from build123d import *

# Parameters (mm, degrees)
F0_R     = 45
F0_R_2   = 30.25
F1_DEPTH = 50
F2_R     = 80
F2_R_2   = 5
F3_DEPTH = 20
F4_R     = 26
F4_R_2   = 21
F5_DEPTH = 30
F6_SIZE2 = 40
F6_SIZE  = 10
F7_R     = 2
F8_DEPTH = 85
F9_R     = 3


with BuildPart() as f1:
    # F0 (on Top) → F1 (new body)
    with BuildSketch(Plane.XY):
        Circle(F0_R)
        Circle(F0_R_2, mode=Mode.SUBTRACT)
    extrude(amount=F1_DEPTH)

    # F2 (on Top) → F3 (join)
    with BuildSketch(Plane.XY):
        Circle(F2_R)
        with Locations((-45, -45)):
            Circle(F2_R_2, mode=Mode.SUBTRACT)
        with Locations((45, -45)):
            Circle(F2_R_2, mode=Mode.SUBTRACT)
        with Locations((-45, 45)):
            Circle(F2_R_2, mode=Mode.SUBTRACT)
        with BuildLine():
            ThreePointArc((40, 45), (45, 50), (50, 45))
            ThreePointArc((50, 45), (45, 40), (40, 45))
        make_face(mode=Mode.SUBTRACT)
    extrude(amount=-F3_DEPTH)

    # F4 (on Top) → F5 (join)
    with BuildSketch(Plane.XY):
        Circle(F4_R)
        Circle(F4_R_2, mode=Mode.SUBTRACT)
    extrude(amount=F5_DEPTH)

    # F6
    f6_edges = [f1.edges().sort_by_distance(p)[0] for p in [
        (-45, 0, 50),
    ]]
    f6_side = f1.faces().sort_by_distance((-43.727208, 0, 50))[0]
    chamfer(f6_edges, length=F6_SIZE, length2=F6_SIZE2, reference=f6_side)

    # F7 (on Front) → F8 (cut, symmetric)
    with BuildSketch(Plane.XZ):
        with BuildLine():
            ThreePointArc((17.5, -6), (19.5, -8), (21.5, -6))
            ThreePointArc((21.5, -6), (19.5, -4), (17.5, -6))
        make_face()
        with Locations((-19.5, -6)):
            Circle(F7_R)
    extrude(amount=F8_DEPTH, both=True, mode=Mode.SUBTRACT)

    # F9
    f9_edges = [f1.edges().sort_by_distance(p)[0] for p in [
        (-80, 0, 0),
    ]]
    fillet(f9_edges, radius=F9_R)


solid = f1.part
Can you work these out from the model? Positions are in its coordinate system, mm. A direction names the side the tool comes from. Coordinates: 2 decimals unless noted, no trailing zeros. Order: outer loops, then holes, each group sorted by start corner. A loop starts at its lowest first (then second) coordinate and runs counter-clockwise, first axis right, second up. Notation, with made-up numbers: M 45,49 L 50,49 A11 ccw 50,65 Z; hole C -5.5,74.25 d11. An arc over 180 degrees is marked long. Answer as CSV lines item,"result".
(1) On a 3-axis mill with a long thin cutter (end or side, diameter ignored), from which of +Z, -Z, +X, -X, +Y, -Y can I reach the whole of each face in a straight line? I mean faces 5 (the cylindrical face through (41, -42, -10)), 6 (the cylindrical face through (20.03, 6.31, 14.79)). Say none if no direction works.
Geometry check:
face 5,"+Z, -Z"
face 6,"+Z"
(2) If we mould it in two halves opening along Z, with no side actions, what happens to faces 1 (the cylindrical face through (41, 42, -10)), 2 (the cylindrical face through (-21.1, -1.1, -7.2)), 3 (the conical face through (36.1, 11.37, 38.61)), 4 (the cylindrical face through (17.9, -1.1, -7.2))? For each: released by +Z, released by -Z, zero draft, split by the parting line, or undercut.
Geometry check:
face 1,"zero draft"
face 2,"undercut"
face 3,"released by +Z"
face 4,"undercut"
(3) Suppose I cut it at D-D on y = -43. Count the separate pieces of the cut face and the enclosed holes in it, plus the area to 3 significant figures.
Geometry check:
separate pieces,"3"
enclosed holes,"2"
area,"2,710 mm^2"
(4) Suppose I cut it at B-B on z = 7.5. Please give me the cut outline in (x, y).
Geometry check:
outline,"C 0,0 d90; C 0,0 d52; hole C 0,0 d60.5; hole C 0,0 d42"
(5) Suppose I cut it at C-C on y = 0. Please give me the cut outline in (x, z), plus the area to 3 significant figures.
Geometry check:
outline,"M -80,-20 L 80,-20 L 80,-3 A3 ccw 77,0 L 45,0 L 45,10 L 35,50 L 30.25,50 L 30.25,0 L 26,0 L 26,30 L 21,30 L 21,0 L -21,0 L -21,30 L -26,30 L -26,0 L -30.25,0 L -30.25,50 L -35,50 L -45,10 L -45,0 L -77,0 A3 ccw -80,-3 Z; hole C -19.5,-6 d4; hole C 19.5,-6 d4"
area,"4,550 mm^2"
(6) Suppose I cut it at A-A on z = -6. Please give me the cut outline in (x, y).
Geometry check:
outline,"M -21.5,-77.06 L -21.5,77.06 A80 ccw Z; M -17.5,-78.06 A80 ccw 17.5,-78.06 L 17.5,78.06 A80 ccw -17.5,78.06 Z; M 21.5,-77.06 A80 ccw 21.5,77.06 Z; hole C -45,-45 d10; hole C -45,45 d10; hole C 45,-45 d10; hole C 45,45 d10"
(7) Please list where these lines run through material, in increasing order: L1, parallel to X at y = -34.5, z = -6; L2, parallel to Y at x = -19, z = 7; L3, parallel to X at y = 8.5, z = 4.
Geometry check:
L1,"-72.18 to -21.5, -17.5 to 17.5, 21.5 to 72.18"
L2,"-40.79 to -23.54, -17.75 to -8.94, 8.94 to 17.75, 23.54 to 40.79"
L3,"-44.19 to -29.03, -24.57 to -19.2, 19.2 to 24.57, 29.03 to 44.19"
(8) I'm going to push flat-ended pins straight in: pin 1 (4.5 mm diameter, centred on x = 19.5, z = -6, fed in from -Y); pin 2 (2 mm diameter, centred on x = -57.5, y = -23.5, fed in from +Z); pin 3 (8 mm diameter, centred on y = -42, z = -10.5, fed in from +X). Where does each tip first touch, or does it pass through?
Geometry check:
pin 1,"y = -78.12"
pin 2,"z = 0"
pin 3,"x = 70.4"
